from build123d import *

# Parameters (mm, degrees)
BOSS_EXTRUDE1_DEPTH     = 30
CUT_EXTRUDE1_START      = -70
SKETCH2_W               = 25
SKETCH2_H               = 30
SKETCH2_W_2             = 5
SKETCH2_H_2             = 10
CUT_EXTRUDE1_DEPTH      = 10
CUT_EXTRUDE2_DEPTH      = 10
CUT_EXTRUDE2_DEPTH_BACK = 10
SKETCH3_R               = 2.5
FILLET1_R               = 1


with BuildPart() as part:
    # Sketch1 → Boss-Extrude1 (new body)
    with BuildSketch(Plane.XY):
        Polygon((-12.5, 70), (12.5, 70), (12.5, -70), (-12.5, -70), (-12.5, 5), (-47.5, 5), (-47.5, 40), (-12.5, 40), align=None)
    extrude(amount=BOSS_EXTRUDE1_DEPTH)

    # Sketch2 → Cut-Extrude1 (cut)
    with BuildSketch(Plane(origin=(0, 0, 0), x_dir=(1, 0, 0), z_dir=(0, 1, 0)).offset(CUT_EXTRUDE1_START)):
        with Locations((0, -15)):
            Rectangle(SKETCH2_W, SKETCH2_H)
        with Locations((0, -15)):
            Rectangle(SKETCH2_W_2, SKETCH2_H_2, mode=Mode.SUBTRACT)
    extrude(amount=CUT_EXTRUDE1_DEPTH, mode=Mode.SUBTRACT)

    # Sketch3 → Cut-Extrude2 (cut, two sides: drawn at the far end of the back side and taken through both)
    with BuildSketch(Plane(origin=(0, 0, 0), x_dir=(0, 0, -1), z_dir=(1, 0, 0)).offset(-CUT_EXTRUDE2_DEPTH_BACK)):
        with Locations(Location((-15, -65, 0), (0, 0, 180))):
            Circle(SKETCH3_R)
    extrude(amount=CUT_EXTRUDE2_DEPTH + CUT_EXTRUDE2_DEPTH_BACK, mode=Mode.SUBTRACT)

    # Fillet1
    fillet1_edges = [part.edges().sort_by_distance(p)[0] for p in [
        (0, -70, 10),
        (0, -70, 20),
    ]]
    fillet(fillet1_edges, radius=FILLET1_R)


solid = part.part
Work out the finished part from the listing and answer in its coordinate system (mm). A direction names the side the tool comes from. Coordinates: 2 decimals unless noted, no trailing zeros. Write each loop counter-clockwise with the first axis right and the second up, starting at its lowest first coordinate (ties: lowest second). Pieces come first, ordered by that corner, then holes.
1. The part is cut by section B-B, the plane y = -65. Write down the section's boundary in (x, z).
Results list:
outline: (-2.5, 10) - (2.5, 10) - (2.5, 12.5) - (-2.5, 12.5) - close; (-2.5, 17.5) - (2.5, 17.5) - (2.5, 20) - (-2.5, 20) - close
2. The part is cut by section D-D, the plane x = -9. Write down the section's boundary in (y, z).
Results list:
outline: (-60, 0) - (70, 0) - (70, 30) - (-60, 30) - close
3. The part is cut by section C-C, the plane z = 2.5. Write down the section's boundary in (x, y).
Results list:
outline: (-47.5, 5) - (-12.5, 5) - (-12.5, -60) - (12.5, -60) - (12.5, 70) - (-12.5, 70) - (-12.5, 40) - (-47.5, 40) - close
4. The part is cut by section A-A, the plane z = 15. Write down the section's boundary in (x, y).
Results list:
outline: (-47.5, 5) - (-12.5, 5) - (-12.5, -60) - (-2.5, -60) - (-2.5, -62.5) - (2.5, -62.5) - (2.5, -60) - (12.5, -60) - (12.5, 70) - (-12.5, 70) - (-12.5, 40) - (-47.5, 40) - close; (-2.5, -70) - (2.5, -70) - (2.5, -67.5) - (-2.5, -67.5) - close
5. For a pull along Z with two mould halves and no side action, classify faces 1 (the flat face through (-10, 6, 30)), 2 (the flat face through (-47.5, 22, 15)), 3 (the cylindrical face through (0, -65.1, 12.5)) as +Z half, -Z half, draft (parallel to the pull), parting line (faces both ways), or undercut.
Results list:
face 1: +Z half
face 2: draft
face 3: undercut
6. For faces 4 (the flat face through (-2.5, -67, 17)), 5 (the flat face through (0, -65, 10)), 6 (the flat face through (-12.5, 55, 15)), determine the directions among +Z, -Z, +X, -X, +Y, -Y from which every point of the face is accessible in a straight line to the end or side of a thin tool.
Results list:
face 4: +Z, -Z, -X, -Y
face 5: -Z, +X, -X, -Y
face 6: +Z, -Z, -X, +Y
7. Flat-ended cylindrical pins translate along their axes: pin 1 (6 mm diameter, centred on y = -65, z = 15, fed in from -X); pin 2 (8 mm diameter, centred on x = -40.5, z = 18, fed in from +Y); pin 3 (9 mm diameter, centred on x = -31, z = 18.5, fed in from -Y). Find the tip coordinate at first contact, or state that the pin passes through.
Results list:
pin 1: stops at x = -2.5
pin 2: stops at y = 40
pin 3: stops at y = 5
8. Consider line 1 along Y through (x, z) = (0.9, 15); line 2 along Y through (x, z) = (1.5, 8.5); line 3 along X through (y, z) = (-26, 10.5). Determine where each line is inside the solid, lowest interval first.
Results list:
line 1: y = -70 to -67.5, -62.5 to 70
line 2: y = -60 to 70
line 3: x = -12.5 to 12.5
